Input: dimensioned drawing with shaded views. Units: mm. Origin: part minimum x, y, z. A direction names the side the tool comes from. Give positions to 0.01 mm unless a question says otherwise; leave off trailing zeros. Order: outer loops, then holes, each group sorted by start corner. A loop starts at its lowest first (then second) coordinate and runs counter-clockwise, first axis right, second up. Notation, with made-up numbers: (50.5, 45) -> (71.5, 45) arc R28 ccw to (71.5, 83) -> close; hole circle Ø10 at (19, -15.5). An arc over 180 degrees is marked (long way). One line per question, with ' | ' between items. Start each with the question number.
(1) Set-up query: the marked faces 4 and 5. Return all of +Z, -Z, +X, -X, +Y, -Y with unobstructed straight access to the full face (end or side cutting, diameter ignored); none if empty.
(2) Section B-B (x = 14.5). Return loops of the section in (y, z) (1 decimal).
(3) First-contact query: pin 1 Ø1 at (y, z) = (12, 1) entering from -X; pin 2 Ø1.5 at (x, z) = (10, 17.5) entering from -Y; pin 3 Ø7 at (y, z) = (16.5, 6.5) entering from +X. Flat tips, straight axial feed; report the tip coordinate or a pass-through.
(4) Mould query, pull axis Y, two halves, no side actions, for the marked faces 1, 2 and 3. Classes: +Y half, -Y half, draft (parallel to the pull), parting line (faces both ways), or undercut.
(5) Section A-A (x = 5.25). Return loops of the section in (y, z) (1 decimal).
(6) Ray query, L1, parallel to X at y = 8.75, z = 20; L2, parallel to Y at x = 15, z = 12; L3, parallel to Y at x = 6.75, z = 11. Return the intervals inside material, ascending.
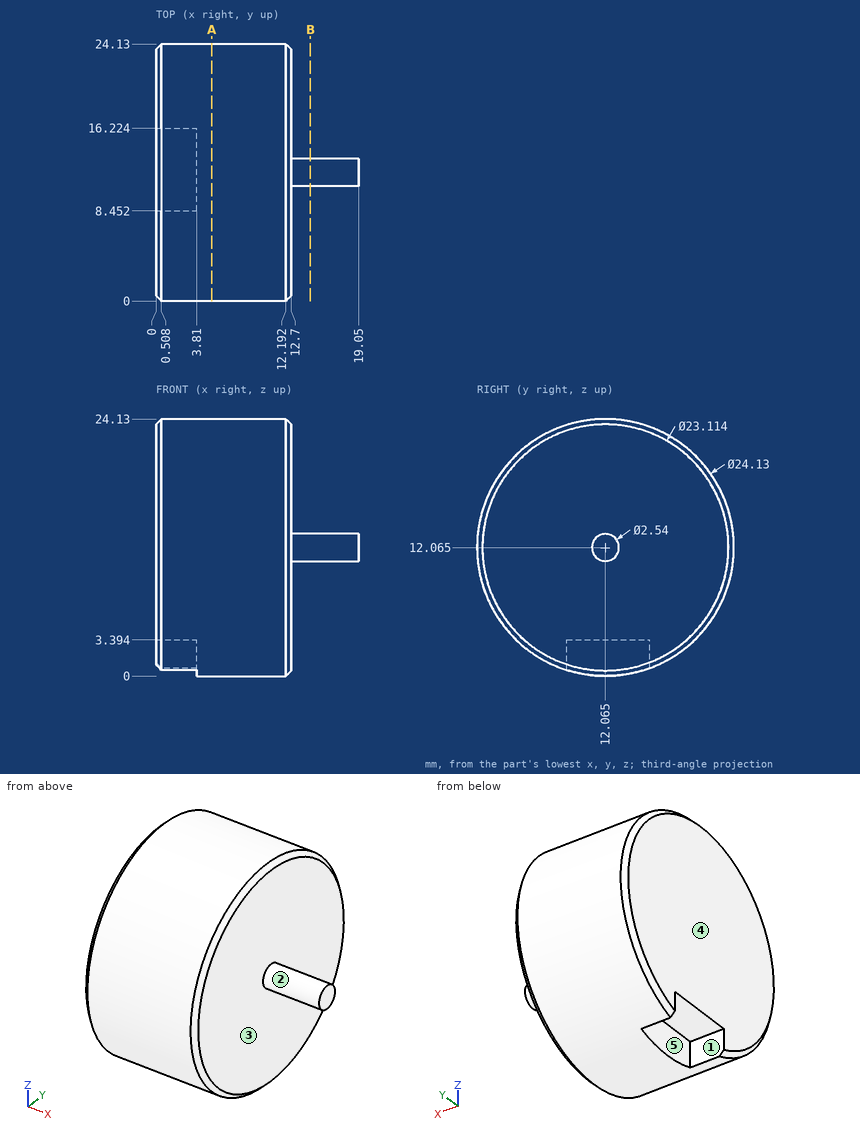
Response:
1) face 4: +Z, -Z, -X, +Y, -Y | face 5: -Z, -X
2) outline: circle Ø2.5 at (12.1, 12.1)
3) pin 1: stops at x = 3.81 | pin 2: stops at y = 0.95 | pin 3: stops at x = 12.7
4) face 1: undercut | face 2: parting line | face 3: draft
5) outline: circle Ø24.1 at (12.1, 12.1)
6) L1: x = 0 to 12.7 | L2: y = 10.8 to 13.33 | L3: y = 0.05 to 24.08
